```python
from build123d import *
from OCP.BRepFilletAPI import BRepFilletAPI_MakeChamfer

# Parameters (mm, degrees)
SKETCH1_R           = 32.5
BOSS_EXTRUDE1_DEPTH = 61.824832
SKETCH2_R           = 20.107463758
CUT_EXTRUDE1_DEPTH  = 78.037717073
CHAMFER1_SIZE       = 2.540972
CHAMFER1_SIZE2      = 1.467031


with BuildPart() as part:
    # Sketch1 → Boss-Extrude1 (new body)
    with BuildSketch(Plane(origin=(0, 0, 0), x_dir=(1, 0, 0), z_dir=(0, 1, 0))):
        with Locations(Location((0, 0, 0), (0, 0, 90))):
            Circle(SKETCH1_R)
    extrude(amount=BOSS_EXTRUDE1_DEPTH)

    # Sketch2 → Cut-Extrude1 (cut, through all)
    with BuildSketch(Plane(origin=(0, 0, 0), x_dir=(1, 0, 0), z_dir=(0, 1, 0))):
        with Locations(Location((0, 0, 0), (0, 0, 90))):
            Circle(SKETCH2_R)
    extrude(amount=CUT_EXTRUDE1_DEPTH, mode=Mode.SUBTRACT)

    # Chamfer1: one chamfer whose edges measure the first distance from different faces: ONE call of the kernel's chamfer builder (chamfer() names one face for all edges)
    chamfer1_edges_1 = [part.edges().sort_by_distance(p)[0] for p in [
        (0, 0, 32.5),
    ]]
    chamfer1_side_1 = [part.faces().sort_by_distance(p)[0] for p in [
        (0, 30.912416, 32.5),
    ]]
    chamfer1_edges_2 = [part.edges().sort_by_distance(p)[0] for p in [
        (0, 61.824832, 32.5),
    ]]
    chamfer1_side_2 = [part.faces().sort_by_distance(p)[0] for p in [
        (0, 61.824832, 31.580761184),
    ]]
    chamfer1_edges_3 = [part.edges().sort_by_distance(p)[0] for p in [
        (0, 0, 20.107463758),
    ]]
    chamfer1_side_3 = [part.faces().sort_by_distance(p)[0] for p in [
        (0, 0, 31.580761184),
    ]]
    chamfer1_edges_4 = [part.edges().sort_by_distance(p)[0] for p in [
        (0, 61.824832, 20.107463758),
    ]]
    chamfer1_side_4 = [part.faces().sort_by_distance(p)[0] for p in [
        (0, 30.912416, 20.107463758),
    ]]
    chamfer1 = BRepFilletAPI_MakeChamfer(part.part.solid().wrapped)
    for e in chamfer1_edges_1:
        chamfer1.Add(CHAMFER1_SIZE, CHAMFER1_SIZE2, e.wrapped, chamfer1_side_1[0].wrapped)  # the first distance lies on this face
    for e in chamfer1_edges_2:
        chamfer1.Add(CHAMFER1_SIZE, CHAMFER1_SIZE2, e.wrapped, chamfer1_side_2[0].wrapped)  # the first distance lies on this face
    for e in chamfer1_edges_3:
        chamfer1.Add(CHAMFER1_SIZE, CHAMFER1_SIZE2, e.wrapped, chamfer1_side_3[0].wrapped)  # the first distance lies on this face
    for e in chamfer1_edges_4:
        chamfer1.Add(CHAMFER1_SIZE, CHAMFER1_SIZE2, e.wrapped, chamfer1_side_4[0].wrapped)  # the first distance lies on this face
    add(Compound.cast(chamfer1.Shape()), mode=Mode.REPLACE)


solid = part.part
```
Design review of the part built by this model. Coordinates are the model's own, in mm. Coordinates: 2 decimals unless noted, no trailing zeros. Order: outer loops, then holes, each group sorted by start corner. A loop starts at its lowest first (then second) coordinate and runs counter-clockwise, first axis right, second up. Notation, with made-up numbers: (87.25, 31.25) - (125.25, 31.25) arc R6 cw to (125.25, 40.25) - close; hole circle Ø1 at (77.25, 65). An arc over 180 degrees is marked (long way). One line per question, with ' | ' between items.
Q1. To check wall thickness, follow line 1 along X through (y, z) = (27, 0); line 2 along Z through (x, y) = (-4.5, 23); line 3 along Z through (x, y) = (-18, 51). State the ranges of each line that lie inside material, in increasing order.
Answer key:
line 1: x = -32.5 to -20.11, 20.11 to 32.5 | line 2: z = -32.19 to -19.6, 19.6 to 32.19 | line 3: z = -27.06 to -8.96, 8.96 to 27.06
Q2. Clearance check with flat-ended pins moving along their axes: pin 1 Ø10 at (y, z) = (27, 2) entering from +X; pin 2 Ø10 at (y, z) = (17.5, 9) entering from +X; pin 3 Ø6 at (y, z) = (33, 8) entering from -X. State where each tip first meets the part, or that it passes through.
Answer key:
pin 1: stops at x = 32.5 | pin 2: stops at x = 32.25 | pin 3: stops at x = -32.11
Q3. Consider section C-C, the plane y = 13.5. Give the boundary of the cut face in (x, z).
Answer key:
outline: circle Ø65 at (0, 0); hole circle Ø40.21 at (0, 0)
Q4. The part is to be moulded in two halves that separate along X. For faces 1 (the conical face through (11.535, 61.733, -27.821)), 2 (the flat face through (23, 0, -2)), 3 (the cylindrical face through (19.63, 29.97, 4.36)), say which applies: +X half, -X half, draft (parallel to the pull), parting line (faces both ways), or undercut.
Answer key:
face 1: parting line | face 2: draft | face 3: undercut
Q5. Consider section B-B, the plane z = 0. Give the boundary of the cut face in (x, y), then the cut area to 3 significant figures.
Answer key:
outline: (-32.5, 2.54) - (-31.03, 0) - (-22.65, 0) - (-20.11, 1.47) - (-20.11, 59.28) - (-21.57, 61.82) - (-29.96, 61.82) - (-32.5, 60.36) - close; (20.11, 1.47) - (22.65, 0) - (31.03, 0) - (32.5, 2.54) - (32.5, 60.36) - (29.96, 61.82) - (21.57, 61.82) - (20.11, 59.28) - close | area: 1,520 mm2
Q6. Consider section A-A, the plane x = 0. Give the boundary of the cut face in (y, z).
Answer key:
outline: (0, -31.03) - (2.54, -32.5) - (60.36, -32.5) - (61.82, -29.96) - (61.82, -21.57) - (59.28, -20.11) - (1.47, -20.11) - (0, -22.65) - close; (0, 22.65) - (1.47, 20.11) - (59.28, 20.11) - (61.82, 21.57) - (61.82, 29.96) - (60.36, 32.5) - (2.54, 32.5) - (0, 31.03) - close
